Input: part model. Units: mm. Frame: model coordinates. Face numbers are marked on the shaded views. A direction names the side the tool comes from. Give positions to 0.01 mm unless a question says otherwise; leave off trailing zeros. Loops run counter-clockwise (first coordinate to the right, second up) from the corner with the lowest first, then second, coordinate; pieces in that order, holes last. Notation, with made-up numbers: (11, 67.25) - (70, 67.25) arc R17 cw to (70, 71.25) - close; hole circle Ø10 at (47, -8.75). An arc over 180 degrees is marked (long way). Answer as a JSON object with one key per item and string values. Group by question number.
(1) Material intervals for L1, parallel to Z at x = 0, y = 10.05; L2, parallel to Y at x = 0, z = 5.5, sorted ascending.
(2) Section query A-A (y = 0). Return loops of the section in (x, z), plus the area to 3 significant figures.
(3) Section query C-C (x = 0). Return loops of the section in (y, z).
(4) Section query B-B (z = 6.5). Return loops of the section in (x, y).
(5) Pin query (flat end, axial travel): P1, Ø4, axis at x = -3, y = -8.5, coming from the -Z side; P2, Ø3.5, axis at x = 0, z = 9, coming from the -Y side; P3, Ø0.9, axis at x = -13.5, z = 6.5, coming from the -Y side; P4, Ø9.5, axis at x = 0, y = 0, coming from the -Z side. Return the tip coordinate at first contact, or that it passes through.
(6) Mould query, pull axis Z, two halves, no side actions, for the marked faces 6, 7 and 8. Classes: +Z half, -Z half, draft (parallel to the pull), parting line (faces both ways), or undercut.
(7) Section query D-D (z = 9). Return loops of the section in (x, y).
(8) Access query for the marked faces 1, 2, 3, 4 and 5. Directions: +Z, -Z, +X, -X, +Y, -Y. A direction counts if a zero-diameter tool reaches every point of the face in a straight line with its end or side. Return the directions, or none.
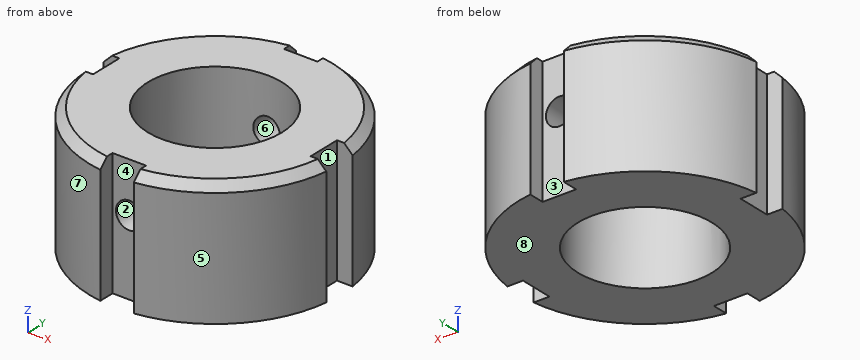
```python
from build123d import *

# Parameters (mm, degrees)
SKETCH1_R           = 15
SKETCH1_R_2         = 8
BOSS_EXTRUDE1_DEPTH = 15
SKETCH2_W           = 4
SKETCH2_H           = 4
CUT_EXTRUDE1_DEPTH  = 26.980762114
CHAMFER1_SIZE       = 1
SKETCH3_R           = 1.600526218
CUT_EXTRUDE2_DEPTH  = 35.964521839


with BuildPart() as part:
    # Sketch1 → Boss-Extrude1 (new body)
    with BuildSketch(Plane.XY):
        Circle(SKETCH1_R)
        Circle(SKETCH1_R_2, mode=Mode.SUBTRACT)
    extrude(amount=BOSS_EXTRUDE1_DEPTH)

    # Sketch2 → Cut-Extrude1 (cut, through all)
    with BuildSketch(Plane.XY.offset(15)):
        with Locations((15, 0)):
            Rectangle(SKETCH2_W, SKETCH2_H)
        with Locations((0, 15)):
            Rectangle(SKETCH2_W, SKETCH2_H)
        with Locations((0, -15)):
            Rectangle(SKETCH2_W, SKETCH2_H)
        with Locations((-15, 0)):
            Rectangle(SKETCH2_W, SKETCH2_H)
    extrude(amount=-CUT_EXTRUDE1_DEPTH, mode=Mode.SUBTRACT)

    # Chamfer1
    chamfer1_edges = [part.edges().sort_by_distance(p)[0] for p in [
        (-10.606601718, 10.606601718, 15),
        (-10.606601718, -10.606601718, 15),
        (10.606601718, -10.606601718, 15),
        (10.606601718, 10.606601718, 15),
    ]]
    chamfer(chamfer1_edges, length=CHAMFER1_SIZE)

    # Sketch3 → Cut-Extrude2 (cut, through all)
    with BuildSketch(Plane(origin=(0, 13, 0), x_dir=(1, 0, 0), z_dir=(0, 1, 0))):
        with Locations(Location((0, -9, 0), (0, 0, 270))):
            Circle(SKETCH3_R)
    extrude(amount=-CUT_EXTRUDE2_DEPTH, mode=Mode.SUBTRACT)


solid = part.part
```
Recorded:
{
 "1": {"L1": "z = 0 to 7.4, 10.6 to 15", "L2": "y = -13 to -8, 8 to 13"},
 "2": {"outline": "(-13, 0) - (-8, 0) - (-8, 15) - (-13, 15) - close; (8, 0) - (13, 0) - (13, 15) - (8, 15) - close", "area": "150 mm^2"},
 "3": {"outline": "(-13, 0) - (-8, 0) - (-8, 7.4) - (-13, 7.4) - close; (-13, 10.6) - (-8, 10.6) - (-8, 15) - (-13, 15) - close; (8, 0) - (13, 0) - (13, 7.4) - (8, 7.4) - close; (8, 10.6) - (13, 10.6) - (13, 15) - (8, 15) - close"},
 "4": {"outline": "(-14.87, -2) arc R15 ccw to (-2, -14.87) - (-2, -13) - (2, -13) - (2, -14.87) arc R15 ccw to (14.87, -2) - (13, -2) - (13, 2) - (14.87, 2) arc R15 ccw to (2, 14.87) - (2, 13) - (-2, 13) - (-2, 14.87) arc R15 ccw to (-14.87, 2) - (-13, 2) - (-13, -2) - close; hole circle Ø16 at (0, 0)"},
 "5": {"P1": "stops at z = 0", "P2": "stops at y = -13", "P3": "stops at y = -7.4", "P4": "passes through"},
 "6": {"face 6": "undercut", "face 7": "draft", "face 8": "-Z half"},
 "7": {"outline": "(-14.87, -2) arc R15 ccw to (-2, -14.87) - (-2, -13) - (-1.6, -13) - (-1.6, -7.84) arc R8 cw to (-1.6, 7.84) - (-1.6, 13) - (-2, 13) - (-2, 14.87) arc R15 ccw to (-14.87, 2) - (-13, 2) - (-13, -2) - close; (1.6, -13) - (2, -13) - (2, -14.87) arc R15 ccw to (14.87, -2) - (13, -2) - (13, 2) - (14.87, 2) arc R15 ccw to (2, 14.87) - (2, 13) - (1.6, 13) - (1.6, 7.84) arc R8 cw to (1.6, -7.84) - close"},
 "8": {"face 1": "+Z, -Z, +X", "face 2": "+Y, -Y", "face 3": "+Z, -Z, +Y", "face 4": "+Z, -Z, -Y", "face 5": "+Z, -Z, +X, -Y"}
}
